Source: CAD feature listing. Evaluate the final solid. Frame: model axes, mm. Face numbers are marked on the shaded views. A direction names the side the tool comes from. Coordinates: 2 decimals unless noted, no trailing zeros. Loops run counter-clockwise (first coordinate to the right, second up) from the corner with the lowest first, then second, coordinate; pieces in that order, holes last. Notation, with made-up numbers: (79, -2) - (114, -2) arc R14 cw to (114, 12) - close; hole circle Ø9 at (78.25, 79.25). An arc over 180 degrees is marked (long way). Use one line per item in the form item = value. Start each with the question number.
Autodesk Fusion 360 part; units mm, degrees
sketch "Sketch1" plane through (0, 0, 0) normal (0, 0, 1) x (1, 0, 0)
  line L0 (18.288, -10.16) -> (-18.288, -10.16)
  line L1 (-18.288, -10.16) -> (-18.288, 10.16)
  line L2 (-18.288, 10.16) -> (18.288, 10.16)
  line L3 (18.288, 10.16) -> (18.288, -10.16)
  line L4 (18.288, -10.16) -> (-18.288, 10.16) construction
  line L5 (-18.288, -10.16) -> (18.288, 10.16) construction
  circle A0 centre (0, 0) radius 2.0574
  dimension "d1" = 36.576
  dimension "d2" = 20.32
  dimension "d3" = 4.1148
extrude "Extrude1" add sketch "Sketch1" along normal blind 6.35
sketch "Sketch2" plane through (0, 0, 6.35) normal (0, 0, 1) x (-1, 0, 0)
  circle A0 centre (0, 0) radius 2.0574
  line L0 (-18.288, -10.16) -> (18.288, -10.16)
  line L1 (18.288, -10.16) -> (18.288, 10.16)
  line L2 (18.288, 10.16) -> (-18.288, 10.16)
  line L3 (-18.288, 10.16) -> (-18.288, -10.16)
  line L4 (18.288, -10.16) -> (13.208, -10.16)
  line L5 (13.208, -10.16) -> (13.208, 10.16)
  line L6 (13.208, 10.16) -> (18.288, 10.16)
  line L7 (18.288, -10.16) -> (18.288, 10.16)
  line L8 (-18.288, -10.16) -> (-13.208, -10.16)
  line L9 (-13.208, -10.16) -> (-13.208, 10.16)
  line L10 (-13.208, 10.16) -> (-18.288, 10.16)
  line L11 (-18.288, -10.16) -> (-18.288, 10.16)
  dimension "d6" = 5.08
  dimension "d7" = 5.08
extrude "Extrude2" add sketch "Sketch2" along normal blind 26.416 contours L0 L2 L3 L8 L9 L10 L11 | L0 L1 L2 L4 L5 L6 L7
sketch "Sketch3" plane through (0, 0, 32.766) normal (0, 0, 1) x (-1, 0, 0)
  line L0 (13.208, -10.16) -> (18.288, -10.16)
  line L1 (18.288, -10.16) -> (18.288, 10.16)
  line L2 (18.288, 10.16) -> (13.208, 10.16)
  line L3 (13.208, 10.16) -> (13.208, -10.16)
  line L4 (18.288, -10.16) -> (-18.288, -10.16)
  line L5 (-18.288, -10.16) -> (-18.288, 10.16)
  line L6 (-18.288, 10.16) -> (18.288, 10.16)
  line L7 (18.288, 10.16) -> (18.288, -10.16)
  point P0 (-18.288, 10.16)
  dimension "d10" = 20.32
  dimension "d11" = 36.576
extrude "Extrude3" add sketch "Sketch3" along normal blind 5.08
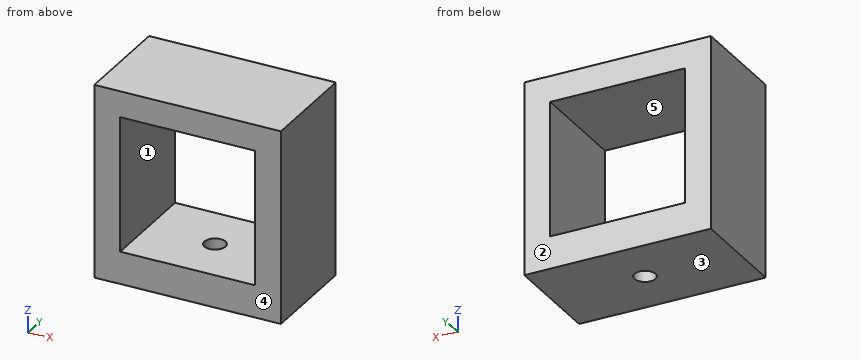
(1) Mould query, pull axis Z, two halves, no side actions, for the marked faces 3, 4 and 5. Classes: +Z half, -Z half, draft (parallel to the pull), parting line (faces both ways), or undercut.
(2) Cut plane B-B, the plane x = 0. Output: boundary loops of the cut face in (y, z).
(3) Cut plane A-A, the plane z = 19. Output: boundary loops of the cut face in (x, y).
(4) Cut plane C-C, the plane x = -10.5. Output: boundary loops of the cut face in (y, z).
(5) Contact query for a flat-ended pin moving along its axis: pin 1 (3.5 mm diameter, centred on x = 0, y = 0, fed in from -Z). Output: stop coordinate, or through.
(6) Cut plane D-D, the plane y = -7.75. Output: boundary loops of the cut face in (x, z), plus the area to 3 significant figures.
(7) Access query for the marked faces 1 and 2. Directions: +Z, -Z, +X, -X, +Y, -Y. A direction counts if a zero-diameter tool reaches every point of the face in a straight line with its end or side. Return the directions, or none.
(8) Material intervals for line 1 (X direction, y = 1.25, z = 16.5); line 2 (Y direction, x = 0, z = 2); line 3 (Z direction, x = 2, y = 1.5), sorted ascending.
Recorded:
q1.face_3 = -Z half
q1.face_4 = draft
q1.face_5 = undercut
q2.outline = (-10.16, 0) - (-2.06, 0) - (-2.06, 6.35) - (-10.16, 6.35) - close; (-10.16, 32.77) - (10.16, 32.77) - (10.16, 37.85) - (-10.16, 37.85) - close; (2.06, 0) - (10.16, 0) - (10.16, 6.35) - (2.06, 6.35) - close
q3.outline = (-18.29, -10.16) - (-13.21, -10.16) - (-13.21, 10.16) - (-18.29, 10.16) - close; (13.21, -10.16) - (18.29, -10.16) - (18.29, 10.16) - (13.21, 10.16) - close
q4.outline = (-10.16, 0) - (10.16, 0) - (10.16, 6.35) - (-10.16, 6.35) - close; (-10.16, 32.77) - (10.16, 32.77) - (10.16, 37.85) - (-10.16, 37.85) - close
q5.pin_1 = 32.77
q6.outline = (-18.29, 0) - (18.29, 0) - (18.29, 37.85) - (-18.29, 37.85) - close; hole (-13.21, 6.35) - (13.21, 6.35) - (13.21, 32.77) - (-13.21, 32.77) - close
q6.area = 686 mm²
q7.face_1 = +Y, -Y
q7.face_2 = +Z, -Z, +X, -X, +Y
q8.line_1 = -18.29 to -13.21, 13.21 to 18.29
q8.line_2 = -10.16 to -2.06, 2.06 to 10.16
q8.line_3 = 0 to 6.35, 32.77 to 37.85
